Geometry: final body of the model. Coordinates: model frame, mm. A direction names the side the tool comes from. Give positions to 0.01 mm unless a question says otherwise; leave off trailing zeros. Loops run counter-clockwise (first coordinate to the right, second up) from the corner with the lowest first, then second, coordinate; pieces in that order, holes last. Notation, with made-up numbers: M -9,-35.75 L 12,-35.75 A17 ccw 12,-7.75 Z; hole C 65.5,18 d8. An arc over 180 degrees is marked long. Put each result on its own line as item: value.
```python
from build123d import *

# Parameters (mm, degrees)
SKETCH1_W           = 61
SKETCH1_H           = 6.1
BOSS_EXTRUDE1_DEPTH = 22.5
SKETCH2_OUTSIDE_W   = 76.06
SKETCH2_OUTSIDE_H   = 21.16
SKETCH2_OUTSIDE_W_2 = 61
SKETCH2_OUTSIDE_H_2 = 5.1952
CUT_EXTRUDE1_DEPTH  = 6
CUT_EXTRUDE3_DEPTH  = 23.5
SKETCH6_R           = 2.4892
CUT_EXTRUDE4_DEPTH  = 7.1
SKETCH7_R           = 1.5
CUT_EXTRUDE5_DEPTH  = 7.1


with BuildPart() as part:
    # Sketch1 → Boss-Extrude1 (new body)
    with BuildSketch(Plane(origin=(0, 0, 0), x_dir=(0, 0, -1), z_dir=(1, 0, 0))):
        with Locations((30.5, 0)):
            Rectangle(SKETCH1_W, SKETCH1_H)
    extrude(amount=BOSS_EXTRUDE1_DEPTH)

    # Sketch2 outside → Cut-Extrude1 (cut)
    with BuildSketch(Plane(origin=(22.5, 0, 0), x_dir=(0, 0, -1), z_dir=(1, 0, 0))):
        with Locations((30.5, 0)):
            Rectangle(SKETCH2_OUTSIDE_W, SKETCH2_OUTSIDE_H)
        with Locations((30.5, 0)):
            Rectangle(SKETCH2_OUTSIDE_W_2, SKETCH2_OUTSIDE_H_2, mode=Mode.SUBTRACT)
    extrude(amount=-CUT_EXTRUDE1_DEPTH, mode=Mode.SUBTRACT)

    # Sketch5 → Cut-Extrude3 (cut, through all)
    with BuildSketch(Plane.ZY):
        with BuildLine():
            Line((-12.3486, -0.1278), (-12.3486, -3.05))
            Line((-12.3486, -3.05), (-17.4134, -3.05))
            Line((-17.4134, -3.05), (-17.4134, -0.1278))
            ThreePointArc((-17.4134, -0.1278), (-14.881, 2.4046), (-12.3486, -0.1278))
        make_face()
    extrude(amount=-CUT_EXTRUDE3_DEPTH, mode=Mode.SUBTRACT)

    # Sketch6 → Cut-Extrude4 (cut, through all)
    with BuildSketch(Plane(origin=(0, 3.05, 0), x_dir=(1, 0, 0), z_dir=(0, 1, 0))):
        with Locations(Location((7.5, 30.5, 0), (0, 0, 270))):  # turned: the seam where the file's is
            Circle(SKETCH6_R)
    extrude(amount=-CUT_EXTRUDE4_DEPTH, mode=Mode.SUBTRACT)

    # Sketch7 → Cut-Extrude5 (cut, through all)
    with BuildSketch(Plane(origin=(0, 3.05, 0), x_dir=(1, 0, 0), z_dir=(0, 1, 0))):
        with Locations(Location((5, 55.5, 0), (0, 0, 270))):  # turned: the seam where the file's is
            Circle(SKETCH7_R)
        with Locations(Location((5, 5.5, 0), (0, 0, 270))):  # turned: the seam where the file's is
            Circle(SKETCH7_R)
    extrude(amount=-CUT_EXTRUDE5_DEPTH, mode=Mode.SUBTRACT)


solid = part.part
```
Item 1: Section C-C on x = 7.5. Output: boundary loops of the cut face in (y, z).
Output values:
outline: M -3.05,-61 L 3.05,-61 L 3.05,-32.99 L -3.05,-32.99 Z; M -3.05,-28.01 L 3.05,-28.01 L 3.05,0 L -3.05,0 L -3.05,-12.35 L -0.13,-12.35 A2.53 cw -0.13,-17.41 L -3.05,-17.41 Z
Item 2: Line query: probe 1 along Z at (x, y) = (3, -1.5); probe 2 along X at (y, z) = (-1.75, -30.5); probe 3 along X at (y, z) = (2.25, -55.5). Output: solid intervals per line, ascending. Write a range as [from, to].
Output values:
probe 1: [-61, -17.41], [-12.35, 0]
probe 2: [0, 5.01], [9.99, 22.5]
probe 3: [0, 3.5], [6.5, 22.5]
Item 3: Set-up query: faces 4 (the flat face through (11, -2, -17.413)), 5 (the flat face through (20, -2.598, -6)), 6 (the flat face through (20, 2.598, -30)). Return all of +Z, -Z, +X, -X, +Y, -Y with unobstructed straight access to the full face (end or side cutting, diameter ignored); none if empty.
Output values:
face 4: +X, -X, -Y
face 5: +Z, -Z, +X, -Y
face 6: +Z, -Z, +X, +Y
Item 4: Section A-A on y = -1.25. Output: boundary loops of the cut face in (x, z).
Output values:
outline: M 0,-61 L 22.5,-61 L 22.5,-17.41 L 0,-17.41 Z; M 0,-12.35 L 22.5,-12.35 L 22.5,0 L 0,0 Z; hole C 5,-55.5 d3; hole C 5,-5.5 d3; hole C 7.5,-30.5 d4.98
Item 5: Mould query, pull axis X, two halves, no side actions, for faces 1 (the flat face through (22.5, 0, -30)), 2 (the cylindrical face through (5.99, 0.04, -32.48)), 3 (the flat face through (20, -2.598, -39)). Classes: pulls with the +X half, pulls with the -X half, needs draft (parallel to the pull), parting line crosses it, or undercut.
Output values:
face 1: pulls with the +X half
face 2: undercut
face 3: needs draft
Item 6: Section B-B on z = -55.5. Output: boundary loops of the cut face in (x, y).
Output values:
outline: M 0,-3.05 L 3.5,-3.05 L 3.5,3.05 L 0,3.05 Z; M 6.5,-3.05 L 16.5,-3.05 L 16.5,-2.6 L 22.5,-2.6 L 22.5,2.6 L 16.5,2.6 L 16.5,3.05 L 6.5,3.05 Z
Item 7: Section D-D on z = -22. Output: boundary loops of the cut face in (x, y).
Output values:
outline: M 0,-3.05 L 16.5,-3.05 L 16.5,-2.6 L 22.5,-2.6 L 22.5,2.6 L 16.5,2.6 L 16.5,3.05 L 0,3.05 Z
Item 8: Pin query (flat end, axial travel): pin 1 Ø1.8 at (x, z) = (5, -55.5) entering from -Y; pin 2 Ø1.8 at (x, z) = (19, -27.5) entering from +Y. Return the tip coordinate at first contact, or that it passes through.
Output values:
pin 1: through
pin 2: y = 2.6
